Geometry check sheet. Reference: the model listing, model coordinates, mm. A direction names the side the tool comes from. Give positions to 0.01 mm unless a question says otherwise; leave off trailing zeros. Loops run counter-clockwise (first coordinate to the right, second up) from the corner with the lowest first, then second, coordinate; pieces in that order, holes last. Notation, with made-up numbers: (81.5, 6) -> (85.5, 6) arc R26 cw to (85.5, 28) -> close; hole circle Ø5 at (54, -11). An arc over 180 degrees is marked (long way). Answer as a JSON object with one key per item and string values.
from build123d import *

# Parameters (mm, degrees)
F0_R     = 10.2
F1_DEPTH = 40
F2_W     = 9.2
F2_H     = 9.2
F3_DEPTH = 20
F4_R     = 16
F4_R_2   = 10.2
F4_W     = 9.2
F4_H     = 9.2
F5_DEPTH = 6
F6_R     = 3


with BuildPart() as f1:
    # F0 (on Top) → F1 (new body)
    with BuildSketch(Plane.XY):
        Circle(F0_R)
    extrude(amount=F1_DEPTH)

    # F2 (on face) → F3 (cut)
    with BuildSketch(Plane.XY.offset(40)):
        Rectangle(F2_W, F2_H)
    extrude(amount=-F3_DEPTH, mode=Mode.SUBTRACT)

    # F4 (on face) → F5 (join)
    with BuildSketch(Plane.XY.offset(40)):
        Circle(F4_R)
        Circle(F4_R_2, mode=Mode.SUBTRACT)
        Circle(F4_R_2)
        Rectangle(F4_W, F4_H, mode=Mode.SUBTRACT)
    extrude(amount=F5_DEPTH)

    # F6
    f6_edges = [f1.edges().sort_by_distance(p)[0] for p in [
        (-16, 0, 46),
    ]]
    fillet(f6_edges, radius=F6_R)


solid = f1.part
1) Section check D-D on z = 12. Record the cut outline in (x, y).
Geometry check:
{"outline": "circle Ø20.4 at (0, 0)"}
2) Draft check along X on faces 4 (the face through (-3.47, -15.62, 41.48)), 5 (the face through (0, 0, 0)), 6 (the face through (4.6, 0, 33)). Enter one of: pulls with the +X half, pulls with the -X half, needs draft (parallel to the pull), parting line crosses it, or undercut.
Geometry check:
{"face 4": "parting line crosses it", "face 5": "needs draft", "face 6": "undercut"}
3) Depth check by flat-ended pin: P1, Ø1, axis at y = 3.5, z = 8, coming from the +X side; P2, Ø2, axis at y = -7.5, z = 36, coming from the +X side; P3, Ø4.5, axis at y = -1.5, z = 39.5, coming from the +X side; P4, Ø10, axis at x = -1.5, z = 27.5, coming from the +Y side. Enter the tip coordinate at first touch or a pass-through.
Geometry check:
{"P1": "stops at x = 9.75", "P2": "stops at x = 7.86", "P3": "stops at x = 16", "P4": "stops at y = 10.2"}
4) Tool access check on faces 1 (the face through (0, -4.6, 33)), 2 (the face through (6, 0, 46)), 3 (the face through (4.707, -9.049, 19.72)). Record the directions out of +Z, -Z, +X, -X, +Y, -Y that give a thin tool (end or side, any length) a straight path to the whole face; none if there is none.
Geometry check:
{"face 1": "+Z", "face 2": "+Z, +X, -X, +Y, -Y", "face 3": "-Z"}
5) Section check B-B on y = 0. Record the cut outline in (x, z).
Geometry check:
{"outline": "(-16, 40) -> (-10.2, 40) -> (-10.2, 0) -> (10.2, 0) -> (10.2, 40) -> (16, 40) -> (16, 43) arc R3 ccw to (13, 46) -> (4.6, 46) -> (4.6, 20) -> (-4.6, 20) -> (-4.6, 46) -> (-13, 46) arc R3 ccw to (-16, 43) -> close"}
6) Section check A-A on z = 36.5. Record the cut outline in (x, y), plus the area to 3 significant figures.
Geometry check:
{"outline": "circle Ø20.4 at (0, 0); hole (-4.6, -4.6) -> (4.6, -4.6) -> (4.6, 4.6) -> (-4.6, 4.6) -> close", "area": "242 mm2"}
7) Material ranges on line 1 along Z through (x, y) = (-7, 9.5); line 2 along X through (y, z) = (2, 30.5); line 3 along Y through (x, z) = (4.5, 44.5), recorded low to high. Write a range as from..to.
Geometry check:
{"line 1": "z = 40..46", "line 2": "x = -10..-4.6, 4.6..10", "line 3": "y = -14.93..-4.6, 4.6..14.93"}
